Here's how the part is built. I have some questions about the finished solid (model axes, mm). A direction names the side the tool comes from. Give positions to 0.01 mm unless a question says otherwise; leave off trailing zeros. Order: outer loops, then holes, each group sorted by start corner. A loop starts at its lowest first (then second) coordinate and runs counter-clockwise, first axis right, second up.
Autodesk Inventor part; units mm, degrees
ref_plane "YZ Plane" through (0, 0, 0) normal (1, 0, 0) x (0, 1, 0)
ref_plane "XZ Plane" through (0, 0, 0) normal (0, 1, 0) x (-1, 0, 0)
ref_plane "XY Plane" through (0, 0, 0) normal (0, 0, 1) x (1, 0, 0)
sketch "Sketch1" plane through (0, 0, 0) normal (0, 1, 0) x (-1, 0, 0)
  circle A0 centre (0, 0) radius 6.3
  dimension "d0" = 12.6
extrude "Extrusion1" add sketch "Sketch1" along normal blind 60
sketch "Sketch2" plane through (0, 0, 0) normal (0, -1, 0) x (1, 0, 0)
  line L0 (-18, 6.5) -> (18, 6.5)
  line L1 (18, 6.5) -> (18, -6.5)
  line L2 (18, -6.5) -> (-18, -6.5)
  line L3 (-18, -6.5) -> (-18, 6.5)
  line L4 (-18, 6.5) -> (18, -6.5) construction
  line L5 (18, 6.5) -> (-18, -6.5) construction
  circle A0 centre (12, 0) radius 1.35
  line L6 (0, 0) -> (0, 6.5) construction
  circle A1 centre (-12, 0) radius 1.35
  dimension "d3" = 2.7
  dimension "d4" = 12
  dimension "d5" = 36
  dimension "d6" = 13
extrude "Extrusion2" add sketch "Sketch2" along normal blind 3
fillet "Fillet1" radius 2 1 edges at (6.3, 0, 0)
fillet "Fillet2" radius 2 4 edges at (-18, -1.5, 6.5) (-18, -1.5, -6.5) (18, -1.5, 6.5) (18, -1.5, -6.5)
sketch "Sketch3" plane through (0, 0, 0) normal (0, 1, 0) x (1, 0, 0)
  circle A0 centre (12, 0) radius 1.35
  line L0 (9.5, 1.4434) -> (12, 2.8868)
  line L1 (12, 2.8868) -> (14.5, 1.4434)
  line L2 (14.5, 1.4434) -> (14.5, -1.4434)
  line L3 (14.5, -1.4434) -> (12, -2.8868)
  line L4 (12, -2.8868) -> (9.5, -1.4434)
  line L5 (9.5, -1.4434) -> (9.5, 1.4434)
  circle A1 centre (-12, 0) radius 1.35
  line L6 (-14.5, 1.4434) -> (-12, 2.8868)
  line L7 (-12, 2.8868) -> (-9.5, 1.4434)
  line L8 (-9.5, 1.4434) -> (-9.5, -1.4434)
  line L9 (-9.5, -1.4434) -> (-12, -2.8868)
  line L10 (-12, -2.8868) -> (-14.5, -1.4434)
  line L11 (-14.5, -1.4434) -> (-14.5, 1.4434)
  line L12 (18, 4.5) -> (18, -4.5)
  line L13 (-18, -4.5) -> (-18, 4.5)
  point P0 (0, 0)
  dimension "d11" = 5
  dimension "d12" = 5
extrude "Extrusion3" cut sketch "Sketch3" against normal blind 1.5
sketch "Sketch4" plane through (0, -3, 0) normal (0, -1, 0) x (1, 0, 0)
  circle A0 centre (-8, -3.5) radius 2.5
  circle A1 centre (-8, 3.5) radius 2.5
  circle A2 centre (-12, 0) radius 1.35
  line L0 (0, 0) -> (0, 6.4158) construction
  circle A3 centre (8, -3.5) radius 2.5
  circle A4 centre (8, 3.5) radius 2.5
  circle A5 centre (12, 0) radius 1.35
  dimension "d15" = 5
  dimension "d16" = 5
  dimension "d17" = 4
  dimension "d18" = 3.5
  dimension "d19" = 4
  dimension "d20" = 3.5
extrude "Extrusion4" cut sketch "Sketch4" against normal blind 2 contours A0 | A1 | A3 | A4
properties part number "PWM3360 holder"
Q1. Thinking about a two-plate mould opening in Z: for faces 1 (the face through (-17.4, -1.52, 5.93)), 2 (the face through (10.767, -0.74, 2.175)), 3 (the face through (-15, 0, 0)), 4 (the face through (17.4, -1.52, -5.93)), which applies, released by +Z, released by -Z, zero draft, split by the parting line, or undercut?
Filled sheet:
face 1: released by +Z
face 2: undercut
face 3: zero draft
face 4: released by -Z
Q2. If we section it at A-A on x = 0: List the corners of the cut face in (y, z) for me.
Filled sheet:
outline: (-3, -6.5) - (1.13, -6.5) arc R2 cw to (2, -6.3) - (60, -6.3) - (60, 6.3) - (2, 6.3) arc R2 cw to (1.13, 6.5) - (-3, 6.5) - close
Q3. I need wall thicknesses on L1, parallel to Z at x = -8, y = -2.3; L2, parallel to X at y = -2.4, z = 0; L3, parallel to Z at x = 12, y = -2.1. Which ranges of each line are inside material? Lowest first, please.
Filled sheet:
L1: z = -6.5 to -6, -1 to 1, 6 to 6.5
L2: x = -18 to -13.35, -10.65 to 10.65, 13.35 to 18
L3: z = -6.5 to -1.35, 1.35 to 6.5
Q4. For faces 5 (the face through (8, -1, -3)), 6 (the face through (-9.5, -1, 0)), 7 (the face through (-10.712, -2.24, -0.406)), which set-ups out of +Z, -Z, +X, -X, +Y, -Y let a thin tool reach every point of the face, with its end or its side?
Filled sheet:
face 5: -Y
face 6: +Y
face 7: +Y, -Y
Q5. If we section it at B-B on y = 18: List the corners of the cut face in (x, z) for me.
Filled sheet:
outline: circle Ø12.6 at (0, 0)
Q6. I'm going to push flat-ended pins straight in: P1, Ø6, axis at y = 38.5, z = 4, coming from the +X side; P2, Ø1.5, axis at x = -8.5, z = -3, coming from the -Y side; P3, Ø1.5, axis at x = 11.5, z = -0.5, coming from the +Y side; P4, Ø2.5, axis at x = -12, z = 0, coming from the +Y side. Where does each tip first touch, or does it pass through?
Filled sheet:
P1: stops at x = 6.22
P2: stops at y = -1
P3: stops at y = -1.5
P4: passes through
